Here's how the part is built. I have some questions about the finished solid (model axes, mm). Round coordinates to 2 decimals unless told otherwise and drop trailing zeros. Loops run counter-clockwise (first coordinate to the right, second up) from the corner with the lowest first, then second, coordinate; pieces in that order, holes last. Notation, with made-up numbers: M -37,75.25 L 11,75.25 A13 cw 11,91.25 Z; hole C -25,31.25 d2. An arc over 180 degrees is marked long. Use a Markdown table: item, result.
Autodesk Inventor part; units mm, degrees
ref_plane "YZ Plane" through (0, 0, 0) normal (1, 0, 0) x (0, 1, 0)
ref_plane "XZ Plane" through (0, 0, 0) normal (0, 1, 0) x (-1, 0, 0)
ref_plane "XY Plane" through (0, 0, 0) normal (0, 0, 1) x (1, 0, 0)
sketch "Sketch2" plane through (0, 0, 0) normal (0, 1, 0) x (-1, 0, 0)
  line L0 (0, 0) -> (-900, 0)
  line L1 (-900, 0) -> (-900, -500)
  line L2 (-900, -500) -> (0, -500)
  line L3 (0, -500) -> (0, 0)
  line L4 (-120, -500) -> (-780, -500)
  line L5 (-780, -500) -> (-780, -463)
  line L6 (-780, -463) -> (-120, -463)
  line L7 (-120, -463) -> (-120, -500)
  line L8 (-120, 0) -> (-780, 0)
  line L9 (-780, 0) -> (-780, -37)
  line L10 (-780, -37) -> (-120, -37)
  line L11 (-120, -37) -> (-120, 0)
  line L12 (-764, -430) -> (-829, -430)
  line L13 (-829, -430) -> (-829, -350)
  line L14 (-829, -350) -> (-764, -350)
  line L15 (-764, -350) -> (-764, -430)
  line L16 (-740, -463) -> (-835, -463)
  line L17 (-835, -463) -> (-835, -430)
  line L18 (-835, -430) -> (-740, -430)
  line L19 (-740, -430) -> (-740, -463)
  line L20 (-740, -430) -> (-764, -350)
  line L21 (-829, -350) -> (-835, -430)
  line L22 (-780, -500) -> (-835, -500)
  line L23 (-835, -500) -> (-835, -463)
  line L24 (-835, -463) -> (-780, -463)
  line L25 (-780, -463) -> (-780, -500)
  line L26 (0, -250) -> (-900, -250)
  line L27 (-829, -150) -> (-764, -150)
  line L28 (-835, -37) -> (-835, -70)
  line L29 (-740, -70) -> (-740, -37)
  line L30 (-740, -70) -> (-764, -150)
  line L31 (-829, -150) -> (-835, -70)
  line L32 (-835, 0) -> (-835, -37)
  point P0 (-780, -463)
  point P1 (-740, -37)
  dimension "d7" = 900
  dimension "d8" = 500
  dimension "d11" = 37
  dimension "d12" = 120
  dimension "d13" = 120
  dimension "d14" = 33
  dimension "d15" = 55
  dimension "d16" = 40
  dimension "d17" = 65
  dimension "d18" = 6
  dimension "d19" = 80
extrude "Extrusion2" add sketch "Sketch2" along normal blind 3 contours L3 L26 L1 L0 L32 L28 L31 L27 L30 L29 L10 L11 | L3 L2 L7 L6 L19 L20 L14 L21 L17 L23 L1 L26
sketch "Sketch3" plane through (0, 3, 0) normal (0, 1, 0) x (1, 0, 0)
  line L0 (0, 500) -> (0, 0)
  line L1 (0, 0) -> (120, 0)
  line L2 (120, 500) -> (0, 500)
  line L3 (900, 0) -> (900, 500)
  point P0 (40, 20)
  point P1 (100, 20)
  point P2 (40, 480)
  point P3 (100, 480)
  point P4 (12.5, 450)
  point P5 (860, 480)
  point P6 (860, 20)
  point P7 (887.5, 450)
  point P8 (12.5, 350)
  point P9 (887.5, 350)
  point P10 (12.5, 250)
  point P11 (887.5, 250)
  point P12 (12.5, 150)
  point P13 (887.5, 150)
  point P14 (12.5, 50)
  point P15 (887.5, 50)
  dimension "d20" = 40
  dimension "d21" = 100
  dimension "d22" = 20
  dimension "d23" = 20
  dimension "d24" = 12.5
  dimension "d25" = 50
  dimension "d33" = 40
  dimension "d34" = 12.5
  dimension "d37" = 100
  dimension "d64" = 50
hole "Hole1" at (40, 3, -20) at (100, 3, -20) at (40, 3, -480) at (100, 3, -480) at (12.5, 3, -450) at (860, 3, -480) at (860, 3, -20) at (887.5, 3, -450) at (12.5, 3, -350) at (887.5, 3, -350) at (12.5, 3, -250) at (887.5, 3, -250) at (12.5, 3, -150) at (887.5, 3, -150) at (12.5, 3, -50) at (887.5, 3, -50) direction (0, -1, 0) diameter 5 end through all
sketch "Sketch4" plane through (0, 0, 0) normal (0, -1, 0) x (1, 0, 0)
  line L0 (120, -37) -> (740, -37)
  line L1 (740, -463) -> (120, -463)
  line L2 (900, 0) -> (900, -500)
  point P0 (0, 0)
  point P1 (630, -447.5)
  point P2 (450, -447.5)
  point P3 (270, -447.5)
  point P4 (270, -52.5)
  point P5 (450, -52.5)
  point P6 (630, -52.5)
  dimension "d49" = 15.5
  dimension "d50" = 15.5
  dimension "d51" = 180
  dimension "d52" = 180
  dimension "d53" = 450
hole "Hole2" at (630, 0, -447.5) at (450, 0, -447.5) at (270, 0, -447.5) at (270, 0, -52.5) at (450, 0, -52.5) at (630, 0, -52.5) direction (0, 1, 0) diameter 5 depth 8 tip angle 118
sketch "Sketch5" plane through (0, 0, 0) normal (0, -1, 0) x (1, 0, 0)
  circle A0 centre (450, -52.5) radius 2.5
  circle A1 centre (270, -447.5) radius 2.5
  circle A2 centre (630, -447.5) radius 2.5
  circle A3 centre (450, -447.5) radius 2.5
  circle A4 centre (270, -52.5) radius 2.5
  circle A5 centre (630, -52.5) radius 2.5
  circle A6 centre (12.5, -50) radius 2.5
  circle A7 centre (12.5, -150) radius 2.5
  circle A8 centre (12.5, -250) radius 2.5
  circle A9 centre (12.5, -350) radius 2.5
  circle A10 centre (860, -20) radius 2.5
  circle A11 centre (12.5, -450) radius 2.5
  circle A12 centre (40, -480) radius 2.5
  circle A13 centre (40, -20) radius 2.5
  circle A14 centre (100, -20) radius 2.5
  circle A15 centre (100, -480) radius 2.5
  circle A16 centre (860, -480) radius 2.5
  circle A17 centre (887.5, -450) radius 2.5
  circle A18 centre (887.5, -350) radius 2.5
  circle A19 centre (887.5, -250) radius 2.5
  circle A20 centre (887.5, -150) radius 2.5
  circle A21 centre (887.5, -50) radius 2.5
  line L0 (835, -430) -> (829, -350)
  line L1 (835, -500) -> (835, -430)
  line L2 (900, -500) -> (835, -500)
  line L3 (900, 0) -> (900, -500)
  line L4 (835, 0) -> (900, 0)
  line L5 (835, -70) -> (835, 0)
  line L6 (829, -150) -> (835, -70)
  line L7 (764, -150) -> (829, -150)
  line L8 (740, -70) -> (764, -150)
  line L9 (740, -37) -> (740, -70)
  line L10 (120, -37) -> (740, -37)
  line L11 (120, 0) -> (120, -37)
  line L12 (0, 0) -> (120, 0)
  line L13 (0, -500) -> (0, 0)
  line L14 (120, -500) -> (0, -500)
  line L15 (120, -463) -> (120, -500)
  line L16 (740, -463) -> (120, -463)
  line L17 (740, -430) -> (740, -463)
  line L18 (764, -350) -> (740, -430)
  line L19 (829, -350) -> (764, -350)
  line L20 (740, -37) -> (740, -70)
  line L21 (740, -37) -> (637, -37)
  line L22 (637, -37) -> (637, -70)
  line L23 (637, -70) -> (740, -70)
  line L24 (740, -70) -> (740, -37)
  line L25 (637, -70) -> (643, -150)
  line L26 (829, -150) -> (835, -70)
  line L27 (764, -150) -> (829, -150)
  line L28 (643, -150) -> (764, -150)
  line L29 (0, -500) -> (0, 0)
  line L30 (0, -250) -> (900, -250)
  line L31 (637, -463) -> (637, -430)
  line L32 (637, -430) -> (643, -350)
  line L33 (643, -350) -> (764, -350)
  dimension "d61" = 103
extrude "Two Motor Cutout" cut sketch "Sketch5" against normal through all contours L31 L32 L33 L18 L17 L16 | L10 L9 L23 L22 | L23 L8 L28 L25
properties part number "Bellypan"
1. Imagine slicing it at B-B, the plane x = 182. Write out the boundary of the cut face in (y, z).
Answer sheet:
| item | result |
|---|---|
| outline | M 0,-463 L 3,-463 L 3,-37 L 0,-37 Z |
2. Imagine slicing it at C-C, the plane y = 1.95. State how many separate pieces and enclosed holes the cut face has, then the cut area to 3 significant figures.
Answer sheet:
| item | result |
|---|---|
| separate pieces | 1 |
| enclosed holes | 22 |
| area | 353,000 mm2 |
3. Imagine slicing it at D-D, the plane z = -123.5. Write out the boundary of the cut face in (x, y).
Answer sheet:
| item | result |
|---|---|
| outline | M 0,0 L 641.01,0 L 641.01,3 L 0,3 Z; M 830.99,0 L 900,0 L 900,3 L 830.99,3 Z |
4. For pin 1 Ø3 at (x, z) = (292, -166) entering from -Y; pin 2 Ø4 at (x, z) = (630, -52.5) entering from -Y; pin 3 Ø1.5 at (x, y) = (585.5, 1.5) entering from +Z; pin 4 Ø1.5 at (x, y) = (412, 1.5) entering from -Z, each with a flat end and sliding along its axis, tell me the tip position at first contact or that it passes through.
Answer sheet:
| item | result |
|---|---|
| pin 1 | y = 0 |
| pin 2 | through |
| pin 3 | z = -37 |
| pin 4 | z = -463 |
5. Imagine slicing it at A-A, the plane z = -386. Write out the boundary of the cut face in (x, y).
Answer sheet:
| item | result |
|---|---|
| outline | M 0,0 L 640.3,0 L 640.3,3 L 0,3 Z; M 831.7,0 L 900,0 L 900,3 L 831.7,3 Z |
6. I need wall thicknesses on probe 1 along Z at (x, y) = (630, 1.15); probe 2 along Z at (x, y) = (12.5, 1.85); probe 3 along X at (y, z) = (1.8, -480). Which ranges of each line are inside material? Lowest first, please. Write a range as from..to.
Answer sheet:
| item | result |
|---|---|
| probe 1 | -463..-450, -445..-55, -50..-37 |
| probe 2 | -500..-452.5, -447.5..-352.5, -347.5..-252.5, -247.5..-152.5, -147.5..-52.5, -47.5..0 |
| probe 3 | 0..37.5, 42.5..97.5, 102.5..120, 835..857.5, 862.5..900 |
